```python
from build123d import *

# Parameters (mm, degrees)
F0_W     = 184.4
F0_H     = 154.5
F0_R     = 11.46558
F1_DEPTH = 4
F2_R     = 5
F3_T     = -1.8
F5_DEPTH = 5.7


with BuildPart() as f1:
    # F0 (on Top) → F1 (new body)
    with BuildSketch(Plane.XY):
        Rectangle(F0_W, F0_H)
        Circle(F0_R, mode=Mode.SUBTRACT)
    extrude(amount=F1_DEPTH)

    # F2
    f2_edges = [f1.edges().sort_by_distance(p)[0] for p in [
        (-92.2, -77.25, 2),
        (-92.2, 77.25, 2),
        (92.2, -77.25, 2),
        (92.2, 77.25, 2),
    ]]
    fillet(f2_edges, radius=F2_R)

    # F3
    f3_openings = [f1.faces().sort_by_distance(p)[0] for p in [
        (0, 74.844307, 4),
    ]]
    offset(amount=F3_T, openings=f3_openings)

    # F4 (on face) → F5 (join)
    with BuildSketch(Plane.XY.offset(1.8)):
        Polygon((-84.4, -39.45), (-84.4, -69.45), (-54.4, -69.45), (-54.4, -67.65), (-82.6, -67.65), (-82.6, -39.45), align=None)
        Polygon((-82.6, 67.65), (-54.4, 67.65), (-54.4, 69.45), (-84.4, 69.45), (-84.4, 39.45), (-82.6, 39.45), align=None)
        Polygon((84.4, -69.45), (84.4, -39.45), (82.6, -39.45), (82.6, -67.65), (54.4, -67.65), (54.4, -69.45), align=None)
        Polygon((82.6, 39.45), (84.4, 39.45), (84.4, 69.45), (54.4, 69.45), (54.4, 67.65), (82.6, 67.65), align=None)
    extrude(amount=F5_DEPTH)


solid = f1.part
```
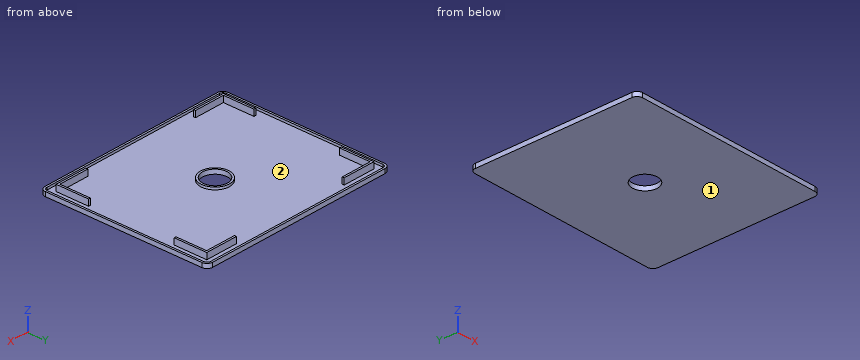
Verification items for the finished model (mm, model axes). Face numbers are marked on the shaded views. Give positions to 0.01 mm unless a question says otherwise; leave off trailing zeros. Loops run counter-clockwise (first coordinate to the right, second up) from the corner with the lowest first, then second, coordinate; pieces in that order, holes last. Notation, with made-up numbers: M 8,-11.5 L 62,-11.5 A7 ccw 62,0.5 Z; hole C 17.5,-29.5 d9. An arc over 180 degrees is marked long. One line per question, with ' | ' between items.
Item 1: Thickness scan on line 1 (Y direction, x = 0, z = 2.15); line 2 (X direction, y = -54.5, z = 2.75); line 3 (Y direction, x = 35, z = 3.5). Record the ranges inside material, lowest first. Write a range as [from, to].
Completed:
line 1: y = [-77.25, -75.45], [-13.27, -11.47], [11.47, 13.27], [75.45, 77.25] | line 2: x = [-92.2, -90.4], [-84.4, -82.6], [82.6, 84.4], [90.4, 92.2] | line 3: y = [-77.25, -75.45], [75.45, 77.25]
Item 2: Section check C-C, the plane x = 60. Record the cut outline in (y, z).
Completed:
outline: M -77.25,0 L 77.25,0 L 77.25,4 L 75.45,4 L 75.45,1.8 L 69.45,1.8 L 69.45,7.5 L 67.65,7.5 L 67.65,1.8 L -67.65,1.8 L -67.65,7.5 L -69.45,7.5 L -69.45,1.8 L -75.45,1.8 L -75.45,4 L -77.25,4 Z
Item 3: Depth check by flat-ended pin: P1, Ø12, axis at x = 64, y = 24, coming from the +Z side; P2, Ø0.9, axis at y = 69, z = 6, coming from the -X side; P3, Ø0.5, axis at x = -84, z = 4.5, coming from the -Y side. Enter the tip coordinate at first touch or a pass-through.
Completed:
P1: stops at z = 1.8 | P2: stops at x = -84.4 | P3: stops at y = -69.45
Item 4: Section check D-D, the plane y = 35.5. Record the cut outline in (x, z), plus the area to 3 significant figures.
Completed:
outline: M -92.2,0 L 92.2,0 L 92.2,4 L 90.4,4 L 90.4,1.8 L -90.4,1.8 L -90.4,4 L -92.2,4 Z | area: 340 mm^2
Item 5: Draft check along Y on the marked faces 1 and 2. Enter one of: +Y half, -Y half, draft (parallel to the pull), parting line (faces both ways), or undercut.
Completed:
face 1: draft | face 2: undercut
Item 6: Section check B-B, the plane y = 0. Record the cut outline in (x, z).
Completed:
outline: M -92.2,0 L -11.47,0 L -11.47,4 L -13.27,4 L -13.27,1.8 L -90.4,1.8 L -90.4,4 L -92.2,4 Z; M 11.47,0 L 92.2,0 L 92.2,4 L 90.4,4 L 90.4,1.8 L 13.27,1.8 L 13.27,4 L 11.47,4 Z
Item 7: Section check A-A, the plane x = 0. Record the cut outline in (y, z), plus the area to 3 significant figures.
Completed:
outline: M -77.25,0 L -11.47,0 L -11.47,4 L -13.27,4 L -13.27,1.8 L -75.45,1.8 L -75.45,4 L -77.25,4 Z; M 11.47,0 L 77.25,0 L 77.25,4 L 75.45,4 L 75.45,1.8 L 13.27,1.8 L 13.27,4 L 11.47,4 Z | area: 253 mm^2
